```python
from build123d import *

# Parameters (mm, degrees)
F_5_0MM_DOWEL_HOLE1_D           = 5
F_5_0MM_DOWEL_HOLE1_DEPTH       = 15
F_5_0MM_DOWEL_HOLE1_CSINK_D     = 5.05
F_5_0MM_DOWEL_HOLE1_CSINK_ANGLE = 90
F_5_0MM_DOWEL_HOLE1_TIP         = 1.502151548
M5_TAPPED_HOLE1_D               = 4.2
M5_TAPPED_HOLE1_DEPTH           = 15
M5_TAPPED_HOLE1_CSINK_D         = 5.05
M5_TAPPED_HOLE1_CSINK_ANGLE     = 90
M5_TAPPED_HOLE1_TIP             = 1.2618073
CUT_EXTRUDE1_DEPTH              = 3
CHAMFER1_SIZE                   = 1
M8_TAPPED_HOLE1_D               = 6.8
M8_TAPPED_HOLE1_DEPTH           = 16
M8_TAPPED_HOLE1_CSINK_D         = 8.05
M8_TAPPED_HOLE1_CSINK_ANGLE     = 90
M8_TAPPED_HOLE1_TIP             = 2.042926105


with BuildPart() as part:
    # Sketch1 → Revolve1 (revolve)
    with BuildSketch(Plane.XY, mode=Mode.PRIVATE) as revolve1_sk:
        Polygon((0, 0), (0, 13), (150, 13), (150, 16), (192, 16), (192, 10), (307, 10), (307, 0), align=None)
    revolve(revolve1_sk.sketch.rotate(Axis((0, 0, 0), (1, 0, 0)), 90), axis=Axis((0, 0, 0), (1, 0, 0)))

    # Ø5.0mm Dowel Hole1
    with Locations(Plane.ZY):
        with Locations((0, 8), (0, -8)):
            CounterSinkHole(F_5_0MM_DOWEL_HOLE1_D / 2, F_5_0MM_DOWEL_HOLE1_CSINK_D / 2, depth=F_5_0MM_DOWEL_HOLE1_DEPTH, counter_sink_angle=F_5_0MM_DOWEL_HOLE1_CSINK_ANGLE)
            with Locations((0, 0, -(F_5_0MM_DOWEL_HOLE1_DEPTH + F_5_0MM_DOWEL_HOLE1_TIP / 2))):  # 118° drill point
                Cone(0, F_5_0MM_DOWEL_HOLE1_D / 2, F_5_0MM_DOWEL_HOLE1_TIP, mode=Mode.SUBTRACT)

    # M5 Tapped Hole1
    with Locations(Plane.ZY):
        with Locations((0, 0)):
            CounterSinkHole(M5_TAPPED_HOLE1_D / 2, M5_TAPPED_HOLE1_CSINK_D / 2, depth=M5_TAPPED_HOLE1_DEPTH, counter_sink_angle=M5_TAPPED_HOLE1_CSINK_ANGLE)
            with Locations((0, 0, -(M5_TAPPED_HOLE1_DEPTH + M5_TAPPED_HOLE1_TIP / 2))):  # 118° drill point
                Cone(0, M5_TAPPED_HOLE1_D / 2, M5_TAPPED_HOLE1_TIP, mode=Mode.SUBTRACT)

    # Sketch7 → Cut-Extrude1 (cut)
    with BuildSketch(Plane.XY.offset(10)):
        with BuildLine():
            Line((307, 2.528133731), (206, 2.528133731))
            ThreePointArc((206, 2.528133731), (203, -0.471866269), (206, -3.471866269))
            Line((206, -3.471866269), (307, -3.471866269))
            Line((307, -3.471866269), (307, 2.528133731))
        make_face()
    extrude(amount=-CUT_EXTRUDE1_DEPTH, mode=Mode.SUBTRACT)

    # Chamfer1
    chamfer1_edges = [part.edges().sort_by_distance(p)[0] for p in [
        (307, 0.494710277, -9.987755591),
        (0, 0, -13),
    ]]
    chamfer(chamfer1_edges, length=CHAMFER1_SIZE)

    # M8 Tapped Hole1
    with Locations(Plane(origin=(307, 0, 0), x_dir=(0, 0, -1), z_dir=(1, 0, 0))):
        with Locations((0, 0)):
            CounterSinkHole(M8_TAPPED_HOLE1_D / 2, M8_TAPPED_HOLE1_CSINK_D / 2, depth=M8_TAPPED_HOLE1_DEPTH, counter_sink_angle=M8_TAPPED_HOLE1_CSINK_ANGLE)
            with Locations((0, 0, -(M8_TAPPED_HOLE1_DEPTH + M8_TAPPED_HOLE1_TIP / 2))):  # 118° drill point
                Cone(0, M8_TAPPED_HOLE1_D / 2, M8_TAPPED_HOLE1_TIP, mode=Mode.SUBTRACT)


solid = part.part
```
The model under review builds one solid part; all positions refer to its coordinate system, in mm. A direction names the side the tool comes from. Round coordinates to 2 decimals unless told otherwise and drop trailing zeros. Order: outer loops, then holes, each group sorted by start corner. A loop starts at its lowest first (then second) coordinate and runs counter-clockwise, first axis right, second up.
(1) Mouldability with a two-part tool opening along Z and no side actions: class faces 1 (the face through (307, -0.1, -4.2)), 2 (the face through (298.58, -3.32, -0.74)), 3 (the face through (171.29, 15.62, -3.47)) as released by +Z, released by -Z, zero draft, split by the parting line, or undercut.
Working result:
face 1: zero draft
face 2: undercut
face 3: split by the parting line
(2) For P1, Ø3, axis at x = 241, z = 8, coming from the -Y side; P2, Ø5, axis at x = 231.5, y = -0.5, coming from the +Z side; P3, Ø8, axis at x = 80.5, y = 8.5, coming from the -Z side, all flat-tipped, find the tip position at first contact; note any pin that passes through.
Working result:
P1: stops at y = -7.6
P2: stops at z = 7
P3: stops at z = -12.2
(3) Take a section at B-B, the plane x = 276. State the section outline as (y, z) points, plus the area to 3 significant figures.
Working result:
outline: (-3.47, 7) - (-3.47, 9.38) arc R10 ccw (long way) to (2.53, 9.68) - (2.53, 7) - close
area: 297 mm2
(4) Take a section at A-A, the plane x = 139.5. State the section outline as (y, z) points.
Working result:
outline: circle Ø26 at (0, 0)
(5) Tool access review of faces 4 (the face through (7.62, -10.44, 0.54)), 5 (the face through (254, 0, 7)), 6 (the face through (250, 6, -8)): name each direction out of +Z, -Z, +X, -X, +Y, -Y from which nothing blocks a thin tool from reaching the whole face with its end or side.
Working result:
face 4: -X
face 5: +Z, +X
face 6: +X
(6) Wall thickness on L1, parallel to Y at x = 3.75, z = 0; L2, parallel to Y at x = 299, z = 0; L3, parallel to Z at x = 295, y = 0: over which ranges is each line inside the solid? List them lowest first.
Working result:
L1: y = -13 to -10.5, -5.5 to -2.1, 2.1 to 5.5, 10.5 to 13
L2: y = -10 to -3.4, 3.4 to 10
L3: z = -10 to -3.4, 3.4 to 7
